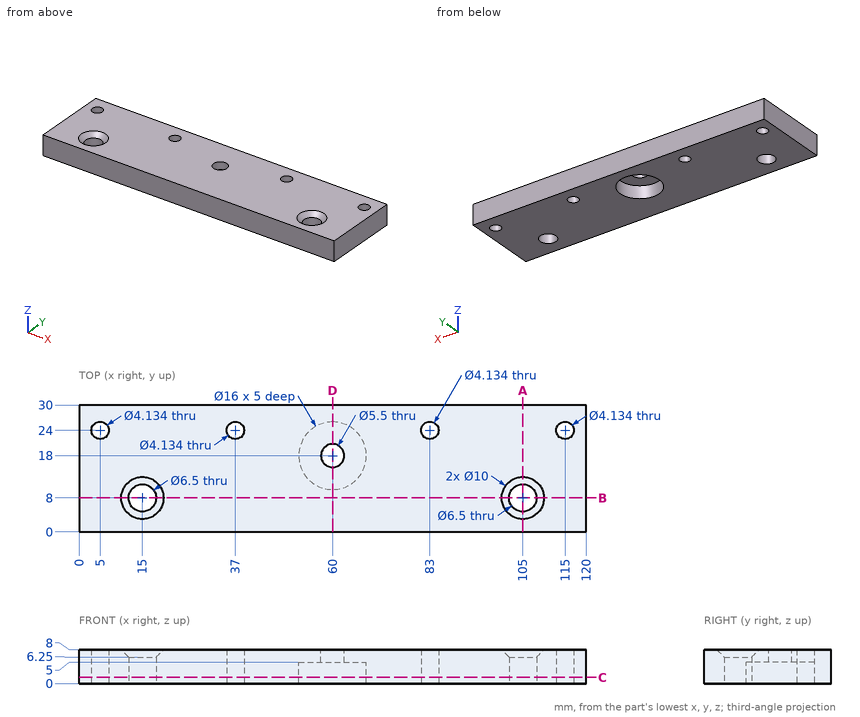
Design review of the part shown in the three views and the two pictorial views. Dimensions are in mm from the part's minimum x, y and z. Coordinates: 2 decimals unless noted, no trailing zeros. Loops run counter-clockwise (first coordinate to the right, second up) from the corner with the lowest first, then second, coordinate; pieces in that order, holes last.
Q1. We need section A-A on x = 105. State the section outline as (y, z) points, and give its area (3 significant figures).
Reported:
outline: (0, 0) - (4.75, 0) - (4.75, 6.25) - (3, 8) - (0, 8) - close; (11.25, 0) - (30, 0) - (30, 8) - (13, 8) - (11.25, 6.25) - close
area: 185 mm2
Q2. We need section B-B on y = 8. State the section outline as (x, z) points.
Reported:
outline: (0, 0) - (11.75, 0) - (11.75, 6.25) - (10, 8) - (0, 8) - close; (18.25, 0) - (101.75, 0) - (101.75, 6.25) - (100, 8) - (20, 8) - (18.25, 6.25) - close; (108.25, 0) - (120, 0) - (120, 8) - (110, 8) - (108.25, 6.25) - close
Q3. We need section D-D on x = 60. State the section outline as (y, z) points.
Reported:
outline: (0, 0) - (10, 0) - (10, 5) - (15.25, 5) - (15.25, 8) - (0, 8) - close; (20.75, 5) - (26, 5) - (26, 0) - (30, 0) - (30, 8) - (20.75, 8) - close
Q4. For pin 1 (5 mm diameter, centred on x = 60.5, y = 20.5, fed in from -Z), flat-tipped, find the tip position at first contact; note if it passes through.
Reported:
pin 1: stops at z = 5
Q5. We need section C-C on z = 1.5. State the section outline as (x, y) points, and give its area (3 significant figures).
Reported:
outline: (0, 0) - (120, 0) - (120, 30) - (0, 30) - close; hole circle Ø4.13 at (5, 24); hole circle Ø6.5 at (15, 8); hole circle Ø4.13 at (37, 24); hole circle Ø16 at (60, 18); hole circle Ø4.13 at (83, 24); hole circle Ø6.5 at (105, 8); hole circle Ø4.13 at (115, 24)
area: 3,280 mm2
Q6. To check wall thickness, follow line 1 (Y direction, x = 15, z = 4.5); line 2 (X direction, y = 24, z = 6.25); line 3 (Y direction, x = 60, z = 3). State the ranges of each line that lie inside material, in increasing order.
Reported:
line 1: y = 0 to 4.75, 11.25 to 30
line 2: x = 0 to 2.93, 7.07 to 34.93, 39.07 to 80.93, 85.07 to 112.93, 117.07 to 120
line 3: y = 0 to 10, 26 to 30
